Design review of the part shown in the three views and the two pictorial views. Dimensions are in mm from the part's minimum x, y and z. Round coordinates to 2 decimals unless told otherwise and drop trailing zeros. Loops run counter-clockwise (first coordinate to the right, second up) from the corner with the lowest first, then second, coordinate; pieces in that order, holes last. Notation, with made-up numbers: M 31,87.25 L 47,87.25 A20 ccw 47,121.25 Z; hole C 35.25,62.25 d1. An arc over 180 degrees is marked long. Return JSON: item names as keys, results as strings. Group by question number.
Q1. Consider section A-A (y = 1.25). State the section outline as (x, z) points, and give its area (3 significant figures).
Q2. Consider section C-C (z = 23). State the section outline as (x, y) points, and give its area (3 significant figures).
Q3. To check wall thickness, follow line 1 along Z through (x, y) = (86.1, 0.9); line 2 along Z through (x, y) = (10.5, 1.6); line 3 along X through (y, z) = (2.15, 23.75). State the ranges of each line that lie inside material, in increasing order.
Q4. Clearance check with a flat-ended pin moving along its axis: pin 1 Ø3.5 at (x, z) = (10.5, 23) entering from +Y. State where the tip first meets the part, or that it passes through.
Q5. Consider section B-B (x = 10.5). State the section outline as (y, z) points.
Q6. Consider section D-D (z = 13.25). State the section outline as (x, y) points, and give its area (3 significant figures).
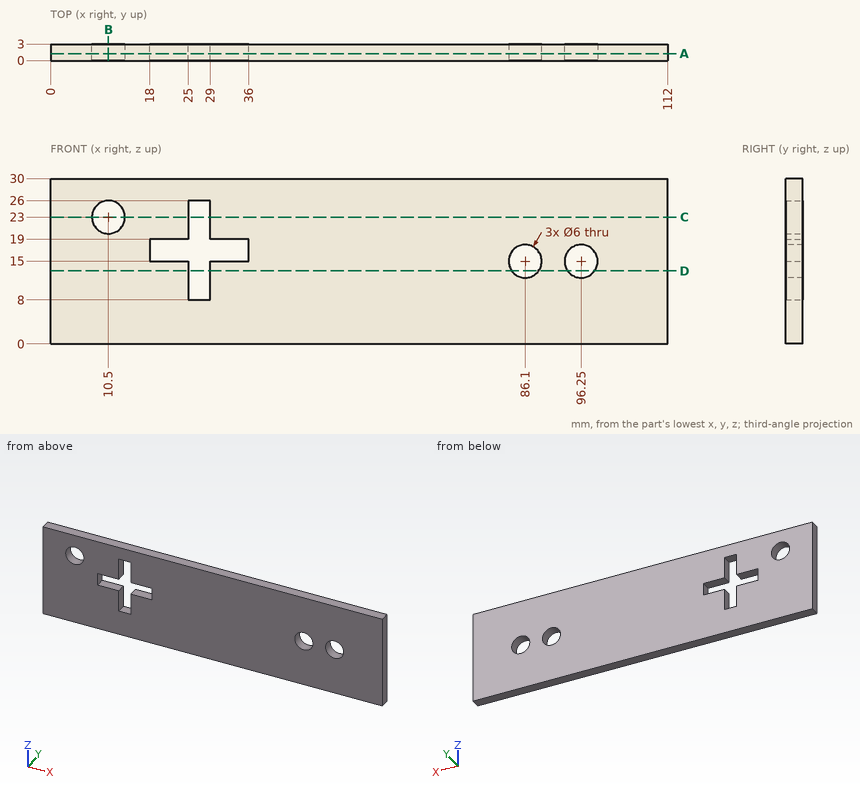
Values:
{
 "1": {"outline": "M 0,0 L 112,0 L 112,30 L 0,30 Z; hole C 10.5,23 d6; hole M 18,15 L 25,15 L 25,8 L 29,8 L 29,15 L 36,15 L 36,19 L 29,19 L 29,26 L 25,26 L 25,19 L 18,19 Z; hole C 86.1,15 d6; hole C 96.25,15 d6", "area": "3,150 mm2"},
 "2": {"outline": "M 0,0 L 7.5,0 L 7.5,3 L 0,3 Z; M 13.5,0 L 25,0 L 25,3 L 13.5,3 Z; M 29,0 L 112,0 L 112,3 L 29,3 Z", "area": "306 mm2"},
 "3": {"line 1": "z = 0 to 12, 18 to 30", "line 2": "z = 0 to 20, 26 to 30", "line 3": "x = 0 to 7.6, 13.4 to 25, 29 to 112"},
 "4": {"pin 1": "passes through"},
 "5": {"outline": "M 0,0 L 3,0 L 3,20 L 0,20 Z; M 0,26 L 3,26 L 3,30 L 0,30 Z"},
 "6": {"outline": "M 0,0 L 25,0 L 25,3 L 0,3 Z; M 29,0 L 83.66,0 L 83.66,3 L 29,3 Z; M 88.54,0 L 93.81,0 L 93.81,3 L 88.54,3 Z; M 98.69,0 L 112,0 L 112,3 L 98.69,3 Z", "area": "295 mm2"}
}
